from build123d import *

# Parameters (mm, degrees)
F0_W     = 15.3987973437
F0_H     = 25.4
F1_DEPTH = 12.7
F3_DEPTH = 12.7


with BuildPart() as f1:
    # F0 (on Front) → F1 (new body)
    with BuildSketch(Plane.XZ):
        Polygon((-27.3676061763, 38.1), (-27.3676061763, 0), (14.38359648, 0), (14.38359648, 25.4), (14.38359648, 38.1), align=None)
        with Locations((22.0829951519, 12.7)):
            Rectangle(F0_W, F0_H)
    extrude(amount=F1_DEPTH)

    # F2 (on Top) → F3 (join)
    with BuildSketch(Plane.XY):
        with BuildLine():
            ThreePointArc((29.7399014235, 19.0850179642), (1.3229484896, 47.2574464843), (-27.0940044443, 19.0850179642))
            Line((-27.0940044443, 19.0850179642), (-11.9244960211, 19.0850179642))
            ThreePointArc((-11.9244960211, 19.0850179642), (1.3229484896, 32.0891530572), (14.5703930003, 19.0850179642))
            Line((14.5703930003, 19.0850179642), (29.7399014235, 19.0850179642))
        make_face()
        with BuildLine():
            ThreePointArc((-27.0940044443, 18.5938467712), (-25.2058095454, 8.6507855756), (-19.9528432558, 0))
            Line((-19.9528432558, 0), (22.598740235, 0))
            ThreePointArc((22.598740235, 0), (27.8517065245, 8.6507855756), (29.7399014235, 18.5938467712))
            Line((29.7399014235, 18.5938467712), (29.7399014235, 19.0850179642))
            Line((29.7399014235, 19.0850179642), (14.5703930003, 19.0850179642))
            ThreePointArc((14.5703930003, 19.0850179642), (14.5721001221, 18.96223044), (14.5726691791, 18.8394323677))
            ThreePointArc((14.5726691791, 18.8394323677), (1.2001504173, 5.5902807351), (-11.9244960211, 19.0850179642))
            Line((-11.9244960211, 19.0850179642), (-27.0940044443, 19.0850179642))
            Line((-27.0940044443, 19.0850179642), (-27.0940044443, 18.5938467712))
        make_face()
        with BuildLine():
            ThreePointArc((29.7399014235, 18.5938467712), (27.8517065245, 8.6507855756), (22.598740235, 0))
            Line((22.598740235, 0), (29.7399014235, 0))
            Line((29.7399014235, 0), (29.7399014235, 18.5938467712))
        make_face()
        with BuildLine():
            Line((-27.0940044443, 18.5938467712), (-27.0940044443, 0))
            Line((-27.0940044443, 0), (-19.9528432558, 0))
            ThreePointArc((-19.9528432558, 0), (-25.2058095454, 8.6507855756), (-27.0940044443, 18.5938467712))
        make_face()
    extrude(amount=F3_DEPTH)


solid = f1.part
The model under review builds one solid part; all positions refer to its coordinate system, in mm. A direction names the side the tool comes from. Give positions to 0.01 mm unless a question says otherwise; leave off trailing zeros. Write each loop counter-clockwise with the first axis right and the second up, starting at its lowest first coordinate (ties: lowest second). Pieces come first, ordered by that corner, then holes. Notation, with made-up numbers: M -1.5,54.5 L 34.5,54.5 A4 ccw 34.5,61.5 Z; hole C 20,32 d6. An arc over 180 degrees is marked long. One line per question, with ' | ' between items. Start each with the question number.
Item 1: For faces 1 (the flat face through (-27.094, 10, 6)), 2 (the flat face through (14, 24, 12.7)), 3 (the flat face through (1, -12.7, 19)), 4 (the flat face through (22, -6, 25.4)), list the 3-axis set-ups (+Z, -Z, +X, -X, +Y, -Y) from which the entire face can be reached by the end or side of a thin tool; tool diameter is ignored.
Item 2: We need section C-C on y = 26. Write out the cut boundary in (x, z).
Item 3: For pin 1 (10 mm diameter, centred on y = -8.5, z = 29, fed in from +X); pin 2 (14 mm diameter, centred on y = 11, z = 8.5, fed in from -X); pin 3 (14 mm diameter, centred on x = 15, y = 17, fed in from +Z); pin 4 (12 mm diameter, centred on x = 3, z = 28.5, fed in from +Y), all flat-tipped, find the tip position at first contact; note any pin that passes through.
Item 4: We need section D-D on z = 34.5. Write out the cut boundary in (x, y), plus the area to 3 significant figures.
Item 5: Wall thickness on line 1 (Z direction, x = -22.5, y = 34); line 2 (Y direction, x = 14.5, z = 22); line 3 (X direction, y = -1, z = 26.5): over which ranges is each line inside the solid? List them lowest first. Write a range as from..to.
Item 6: We need section B-B on x = 7. Write out the cut boundary in (y, z), plus the area to 3 significant figures.
Results found:
1) face 1: +Z, -Z, -X, +Y | face 2: +Z, +X, -X, +Y | face 3: +Z, -Z, +X, -X, -Y | face 4: +Z, +X, +Y, -Y
2) outline: M -26.18,0 L -9.83,0 L -9.83,12.7 L -26.18,12.7 Z; M 12.47,0 L 28.82,0 L 28.82,12.7 L 12.47,12.7 Z
3) pin 1: stops at x = 29.78 | pin 2: stops at x = -27.09 | pin 3: stops at z = 12.7 | pin 4: stops at y = 0
4) outline: M -27.37,-12.7 L 14.38,-12.7 L 14.38,0 L -27.37,0 Z | area: 530 mm2
5) line 1: z = 0..12.7 | line 2: y = -12.7..0 | line 3: x = -27.37..14.38
6) outline: M -12.7,0 L 6.87,0 L 6.87,12.7 L 0,12.7 L 0,38.1 L -12.7,38.1 Z; M 30.81,0 L 46.68,0 L 46.68,12.7 L 30.81,12.7 Z | area: 773 mm2
